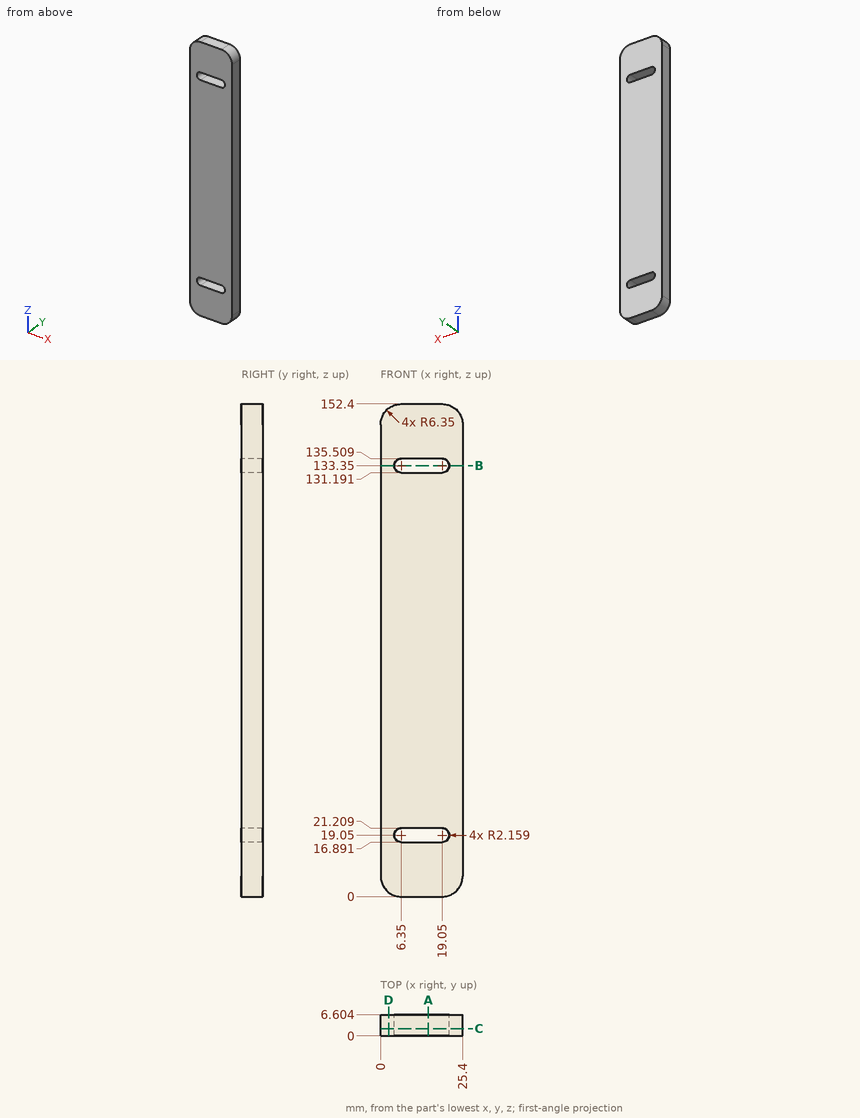
Print and shaded views of the part. All mm, measured from the part's lowest x, y and z. Coordinates: 2 decimals unless noted, no trailing zeros. Order: outer loops, then holes, each group sorted by start corner. A loop starts at its lowest first (then second) coordinate and runs counter-clockwise, first axis right, second up.
Item 1: Drop a flat-ended pin along its axis: pin 1 Ø10 at (x, z) = (6.5, 107.5) entering from -Y. Give the stop position or say it passes through.
Filled in:
pin 1: stops at y = 0
Item 2: Saw through at B-B on z = 133.35. List the corners of the cut face in (x, y).
Filled in:
outline: (0, 0) - (4.19, 0) - (4.19, 6.6) - (0, 6.6) - close; (21.21, 0) - (25.4, 0) - (25.4, 6.6) - (21.21, 6.6) - close
Item 3: Drill centre lines: L1, parallel to Z at x = 8.25, y = 5.75; L2, parallel to Z at x = 19.75, y = 2.75; L3, parallel to Z at x = 4, y = 3. Where is each one in solid material? Low to high.
Filled in:
L1: z = 0 to 16.89, 21.21 to 131.19, 135.51 to 152.4
L2: z = 0.04 to 17.01, 21.09 to 131.31, 135.39 to 152.36
L3: z = 0.45 to 151.95
Item 4: Saw through at C-C on y = 2.25. List the corners of the cut face in (x, z).
Filled in:
outline: (0, 6.35) arc R6.35 ccw to (6.35, 0) - (19.05, 0) arc R6.35 ccw to (25.4, 6.35) - (25.4, 146.05) arc R6.35 ccw to (19.05, 152.4) - (6.35, 152.4) arc R6.35 ccw to (0, 146.05) - close; hole (6.35, 16.89) - (19.05, 16.89) arc R2.16 ccw to (19.05, 21.21) - (6.35, 21.21) arc R2.16 ccw to start; hole (6.35, 131.19) - (19.05, 131.19) arc R2.16 ccw to (19.05, 135.51) - (6.35, 135.51) arc R2.16 ccw to start
Item 5: Saw through at A-A on x = 14.75. List the corners of the cut face in (y, z).
Filled in:
outline: (0, 0) - (6.6, 0) - (6.6, 16.89) - (0, 16.89) - close; (0, 21.21) - (6.6, 21.21) - (6.6, 131.19) - (0, 131.19) - close; (0, 135.51) - (6.6, 135.51) - (6.6, 152.4) - (0, 152.4) - close
Item 6: Saw through at D-D on x = 2.5. List the corners of the cut face in (y, z), then the cut area to 3 significant figures.
Filled in:
outline: (0, 1.3) - (6.6, 1.3) - (6.6, 151.1) - (0, 151.1) - close
area: 989 mm2
